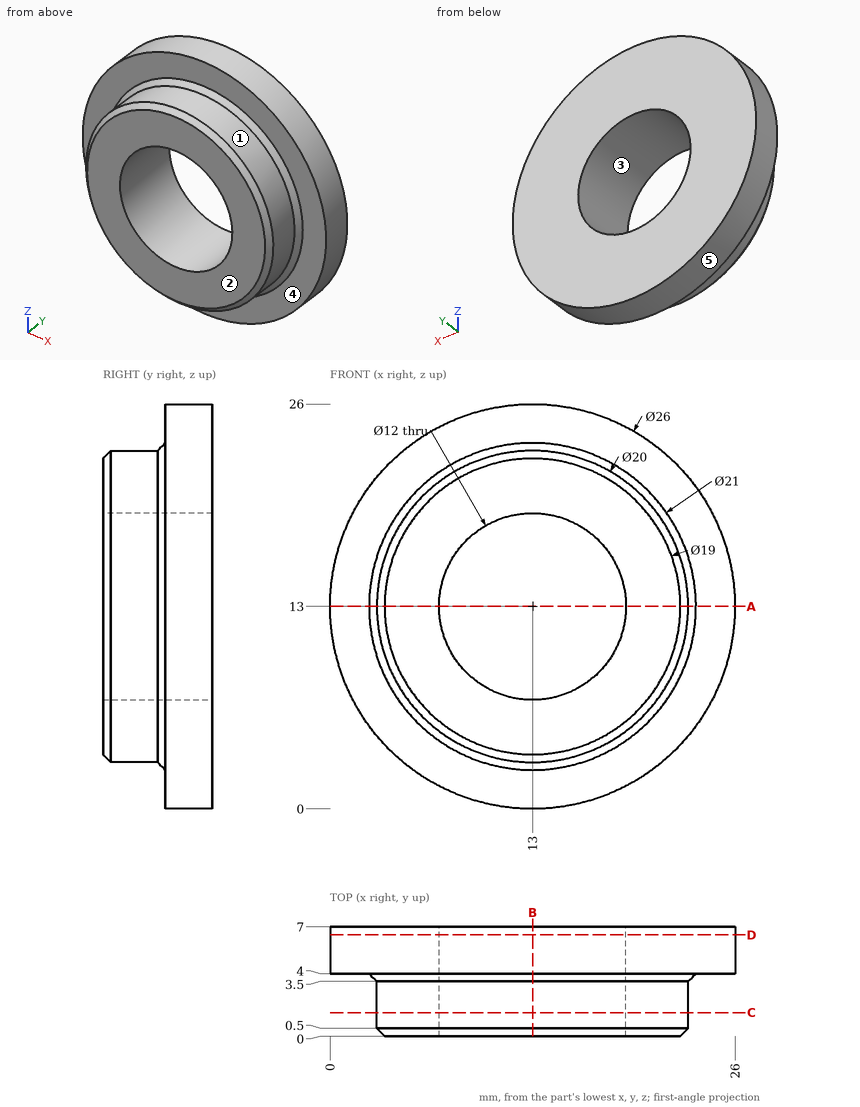
Answer from the drawing. Dimensions are ordinates in mm from the lowest x, y and z of the part. A direction names the side the tool comes from. Coordinates: 2 decimals unless noted, no trailing zeros. Loops run counter-clockwise (first coordinate to the right, second up) from the corner with the lowest first, then second, coordinate; pieces in that order, holes last. Notation, with made-up numbers: (42, 5) -> (98, 5) arc R20 cw to (98, 11) -> close; hole circle Ø2 at (49.25, -5). An arc over 180 degrees is marked (long way). Return JSON: item names as keys, results as strings.
Item 1: Find section C-C (y = 1.5). Determine the outline of the cut face in (x, z), plus the area to 3 significant figures.
Answers:
{"outline": "circle Ø20 at (13, 13); hole circle Ø12 at (13, 13)", "area": "201 mm2"}
Item 2: Flat-ended cylindrical pins translate along their axes: P1, Ø2, axis at y = 1.5, z = 3, coming from the +X side; P2, Ø4, axis at x = 6, y = 1, coming from the +Z side; P3, Ø1, axis at y = 3, z = 15, coming from the -X side; P4, Ø4, axis at x = 10, z = 7.5, coming from the -Y side. Find the tip coordinate at first contact, or state that the pin passes through.
Answers:
{"P1": "stops at x = 17.36", "P2": "stops at z = 21.66", "P3": "stops at x = 3.11", "P4": "stops at y = 0"}
Item 3: Find section A-A (z = 13). Determine the outline of the cut face in (x, y), plus the area to 3 significant figures.
Answers:
{"outline": "(0, 4) -> (2.5, 4) -> (3, 3.5) -> (3, 0.5) -> (3.5, 0) -> (7, 0) -> (7, 7) -> (0, 7) -> close; (19, 0) -> (22.5, 0) -> (23, 0.5) -> (23, 3.5) -> (23.5, 4) -> (26, 4) -> (26, 7) -> (19, 7) -> close", "area": "74.0 mm2"}
Item 4: For a pull along Z with two mould halves and no side action, classify the marked faces 1, 2 and 3 as +Z half, -Z half, draft (parallel to the pull), parting line (faces both ways), or undercut.
Answers:
{"face 1": "parting line", "face 2": "draft", "face 3": "undercut"}
Item 5: For the marked faces 4 and 5, determine the directions among +Z, -Z, +X, -X, +Y, -Y from which every point of the face is accessible in a straight line to the end or side of a thin tool.
Answers:
{"face 4": "-Y", "face 5": "+Y, -Y"}
Item 6: Find the intervals of material crossed by probe 1 along X at (y, z) = (4.5, 13); probe 2 along X at (y, z) = (3.5, 13); probe 3 along Z at (x, y) = (15.5, 2.5), in increasing order.
Answers:
{"probe 1": "x = 0 to 7, 19 to 26", "probe 2": "x = 3 to 7, 19 to 23", "probe 3": "z = 3.32 to 7.55, 18.45 to 22.68"}
Item 7: Find section B-B (x = 13). Determine the outline of the cut face in (y, z).
Answers:
{"outline": "(0, 3.5) -> (0.5, 3) -> (3.5, 3) -> (4, 2.5) -> (4, 0) -> (7, 0) -> (7, 7) -> (0, 7) -> close; (0, 19) -> (7, 19) -> (7, 26) -> (4, 26) -> (4, 23.5) -> (3.5, 23) -> (0.5, 23) -> (0, 22.5) -> close"}
Item 8: Find section D-D (y = 6.5). Determine the outline of the cut face in (x, z), plus the area to 3 significant figures.
Answers:
{"outline": "circle Ø26 at (13, 13); hole circle Ø12 at (13, 13)", "area": "418 mm2"}
